The model under review builds one solid part; all positions refer to its coordinate system, in mm. Round coordinates to 2 decimals unless told otherwise and drop trailing zeros. Order: outer loops, then holes, each group sorted by start corner. A loop starts at its lowest first (then second) coordinate and runs counter-clockwise, first axis right, second up. Notation, with made-up numbers: M 13,34 L 34,34 A28 ccw 34,67 Z; hole C 20,48 d7. An arc over 180 degrees is marked long. One line per item, written item: value. Start each with the question number.
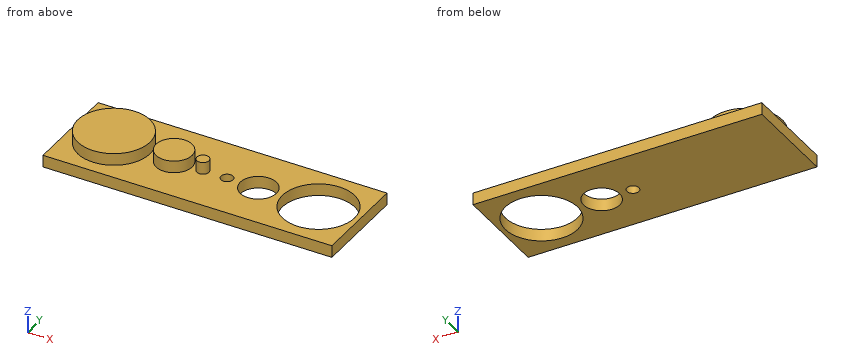
from build123d import *

# Parameters (mm, degrees)
F0_W     = 120
F0_H     = 40
F0_R     = 2.5
F0_R_2   = 7.5
F0_R_3   = 15
F1_DEPTH = 5
F2_R     = 2.5
F2_R_2   = 7.5
F2_R_3   = 15
F3_DEPTH = 5


with BuildPart() as f1:
    # F0 (on Top) → F1 (new body)
    with BuildSketch(Plane.XY):
        Rectangle(F0_W, F0_H)
        with Locations((5, 0)):
            Circle(F0_R, mode=Mode.SUBTRACT)
        with Locations((18, 0)):
            Circle(F0_R_2, mode=Mode.SUBTRACT)
        with Locations((43, 0)):
            Circle(F0_R_3, mode=Mode.SUBTRACT)
    extrude(amount=F1_DEPTH)

    # F2 (on face) → F3 (join)
    with BuildSketch(Plane.XY.offset(5)):
        with Locations((-5, 0)):
            Circle(F2_R)
        with Locations((-17, 0)):
            Circle(F2_R_2)
        with Locations((-42, 0)):
            Circle(F2_R_3)
    extrude(amount=F3_DEPTH)


solid = f1.part
Item 1: Consider section D-D, the plane z = 2.5. Give the boundary of the cut face in (x, y), then the cut area to 3 significant figures.
Item 2: Consider section A-A, the plane x = 43. Give the boundary of the cut face in (y, z).
Item 3: Consider section B-B, the plane y = 5. Give the boundary of the cut face in (x, z).
Item 4: Consider section C-C, the plane x = -17. Give the boundary of the cut face in (y, z).
Item 5: Wall thickness on L1, parallel to Y at x = 43, z = 2.4; L2, parallel to Y at x = 18, z = 2.55; L3, parallel to X at y = 0.5, z = 1: over which ranges is each line inside the solid? List them lowest first.
Item 6: Clearance check with flat-ended pins moving along their axes: P1, Ø12, axis at x = -9.5, y = -1.5, coming from the -Z side; P2, Ø1, axis at y = 6, z = 7, coming from the -X side. State where each tip first meets the part, or that it passes through.
Computed:
1. outline: M -60,-20 L 60,-20 L 60,20 L -60,20 Z; hole C 5,0 d5; hole C 18,0 d15; hole C 43,0 d30
1. area: 3,900 mm^2
2. outline: M -20,0 L -15,0 L -15,5 L -20,5 Z; M 15,0 L 20,0 L 20,5 L 15,5 Z
3. outline: M -60,0 L 12.41,0 L 12.41,5 L -11.41,5 L -11.41,10 L -22.59,10 L -22.59,5 L -27.86,5 L -27.86,10 L -56.14,10 L -56.14,5 L -60,5 Z; M 23.59,0 L 28.86,0 L 28.86,5 L 23.59,5 Z; M 57.14,0 L 60,0 L 60,5 L 57.14,5 Z
4. outline: M -20,0 L 20,0 L 20,5 L 7.5,5 L 7.5,10 L -7.5,10 L -7.5,5 L -20,5 Z
5. L1: y = -20 to -15, 15 to 20
5. L2: y = -20 to -7.5, 7.5 to 20
5. L3: x = -60 to 2.55, 7.45 to 10.52, 25.48 to 28.01, 57.99 to 60
6. P1: stops at z = 0
6. P2: stops at x = -55.96
